```python
from build123d import *

# Parameters (mm, degrees)
SKETCH1_R           = 3.556
BOSS_EXTRUDE3_DEPTH = 25.4
CUT_EXTRUDE3_DEPTH  = 23.8125


with BuildPart() as part:
    # Sketch1 → Boss-Extrude3 (new body)
    with BuildSketch(Plane(origin=(0, 0, 0), x_dir=(1, 0, 0), z_dir=(0, 1, 0))):
        with BuildLine():
            Line((-136.525, -12.7), (136.525, -12.7))
            ThreePointArc((136.525, -12.7), (138.77006403, -11.77006403), (139.7, -9.525))
            Line((139.7, -9.525), (139.7, 9.525))
            ThreePointArc((139.7, 9.525), (138.77006403, 11.77006403), (136.525, 12.7))
            Line((136.525, 12.7), (-136.525, 12.7))
            ThreePointArc((-136.525, 12.7), (-138.77006403, 11.77006403), (-139.7, 9.525))
            Line((-139.7, 9.525), (-139.7, -9.525))
            ThreePointArc((-139.7, -9.525), (-138.77006403, -11.77006403), (-136.525, -12.7))
        make_face()
        with Locations((127, 0)):
            Circle(SKETCH1_R, mode=Mode.SUBTRACT)
        with Locations((-127, 0)):
            Circle(SKETCH1_R, mode=Mode.SUBTRACT)
    extrude(amount=BOSS_EXTRUDE3_DEPTH)

    # Sketch5 → Cut-Extrude3 (cut)
    with BuildSketch(Plane.XZ):
        with BuildLine():
            Line((-136.525, 11.1125), (-136.525, 12.7))
            Line((-136.525, 12.7), (-111.125, 12.7))
            Line((-111.125, 12.7), (-111.125, 11.1125))
            Line((-111.125, 11.1125), (111.125, 11.1125))
            Line((111.125, 11.1125), (111.125, 12.7))
            Line((111.125, 12.7), (136.525, 12.7))
            Line((136.525, 12.7), (136.525, 11.1125))
            ThreePointArc((136.525, 11.1125), (137.647532015, 10.647532015), (138.1125, 9.525))
            Line((138.1125, 9.525), (138.1125, -9.525))
            ThreePointArc((138.1125, -9.525), (137.647532015, -10.647532015), (136.525, -11.1125))
            Line((136.525, -11.1125), (-136.525, -11.1125))
            ThreePointArc((-136.525, -11.1125), (-137.647532015, -10.647532015), (-138.1125, -9.525))
            Line((-138.1125, -9.525), (-138.1125, 9.525))
            ThreePointArc((-138.1125, 9.525), (-137.647532015, 10.647532015), (-136.525, 11.1125))
        make_face()
    extrude(amount=-CUT_EXTRUDE3_DEPTH, mode=Mode.SUBTRACT)


solid = part.part
```
Check sheet for the modelled part. Datum: model origin and axes. Units: mm. A direction names the side the tool comes from. Give positions to 0.01 mm unless a question says otherwise; leave off trailing zeros. Order: outer loops, then holes, each group sorted by start corner. A loop starts at its lowest first (then second) coordinate and runs counter-clockwise, first axis right, second up. Notation, with made-up numbers: M 46.5,55.25 L 63.5,55.25 A36 ccw 63.5,89.25 Z; hole C 47.25,-23 d1. An arc over 180 degrees is marked long. Answer in a Markdown table with one row per item. Add a question column.
Q1. Sectioned sample at B-B, the plane z = 0. Record the boundary of the cut face in (x, y).
Q2. Sectioned sample at D-D, the plane x = 56. Record the boundary of the cut face in (y, z), and give its area (3 significant figures).
Q3. Sectioned sample at A-A, the plane x = -127. Record the boundary of the cut face in (y, z).
Q4. Release check for a two-part mould opening along Z. For faces 1 (the flat face through (2, 12, -11.112)), 2 (the flat face through (2, 13, -12.7)), 3 (the flat face through (139.7, 13, 0)) record: released by +Z, released by -Z, zero draft, split by the parting line, or undercut.
Q5. Access from +Z, -Z, +X, -X, +Y, -Y to the whole of each face (thin tool, end or side, straight path). Record for faces 4 (the flat face through (138.112, 12, 0)), 5 (the flat face through (-2, 13, 12.7)).
Q6. Gauge pin test, flat ends, axial feed: pin 1 Ø5.5 at (x, z) = (-127, 0) entering from +Y; pin 2 Ø1.7 at (y, z) = (7.5, 12) entering from +X; pin 3 Ø1.3 at (y, z) = (17, 12) entering from +X; pin 4 Ø1.7 at (y, z) = (17.5, 12) entering from -X. Record the tip position at first contact, or that the pin passes through.
Q7. Thickness scan on L1, parallel to X at y = 24.9, z = 0; L2, parallel to Z at x = 69.5, y = 11.5; L3, parallel to Z at x = -127, y = 24.75. Record the ranges inside material, lowest first.
Verdict:
| question | item | result |
|---|---|---|
| 1 | outline | M -139.7,0 L -138.11,0 L -138.11,23.81 L -130.56,23.81 L -130.56,25.4 L -139.7,25.4 Z; M -123.44,23.81 L 123.44,23.81 L 123.44,25.4 L -123.44,25.4 Z; M 130.56,23.81 L 138.11,23.81 L 138.11,0 L 139.7,0 L 139.7,25.4 L 130.56,25.4 Z |
| 2 | outline | M 0,-12.7 L 25.4,-12.7 L 25.4,12.7 L 0,12.7 L 0,11.11 L 23.81,11.11 L 23.81,-11.11 L 0,-11.11 Z |
| 2 | area | 116 mm² |
| 3 | outline | M 0,-12.7 L 25.4,-12.7 L 25.4,-3.56 L 23.81,-3.56 L 23.81,-11.11 L 0,-11.11 Z; M 23.81,3.56 L 25.4,3.56 L 25.4,12.7 L 23.81,12.7 Z |
| 4 | face 1 | undercut |
| 4 | face 2 | released by -Z |
| 4 | face 3 | zero draft |
| 5 | face 4 | -Y |
| 5 | face 5 | +Z, +X, -X, +Y, -Y |
| 6 | pin 1 | through |
| 6 | pin 2 | x = 139.25 |
| 6 | pin 3 | x = 139.12 |
| 6 | pin 4 | x = -139.25 |
| 7 | L1 | -139.7 to -130.56, -123.44 to 123.44, 130.56 to 139.7 |
| 7 | L2 | -12.7 to -11.11, 11.11 to 12.7 |
| 7 | L3 | -12.7 to -3.56, 3.56 to 12.7 |
